from build123d import *

# Parameters (mm, degrees)
SKETCH1_W           = 84
SKETCH1_H           = 50.8
SKETCH1_R           = 2.1
BOSS_EXTRUDE1_DEPTH = 6
SKETCH3_W           = 20
SKETCH3_H           = 50.8
BOSS_EXTRUDE2_DEPTH = 20
SKETCH5_R           = 6.5
CUT_EXTRUDE1_DEPTH  = 10
CUT_EXTRUDE2_START  = -10
SKETCH6_R           = 6.5
CUT_EXTRUDE2_DEPTH  = 10
SKETCH7_W           = 10
SKETCH7_H           = 15
CUT_EXTRUDE3_DEPTH  = 10


with BuildPart() as part:
    # Sketch1 → Boss-Extrude1 (new body)
    with BuildSketch(Plane.XY):
        with Locations((42, 25.4)):
            Rectangle(SKETCH1_W, SKETCH1_H)
        with Locations((72, 39.4)):
            Circle(SKETCH1_R, mode=Mode.SUBTRACT)
        with Locations((72, 11.4)):
            Circle(SKETCH1_R, mode=Mode.SUBTRACT)
        with Locations((44, 39.4)):
            Circle(SKETCH1_R, mode=Mode.SUBTRACT)
        with Locations((44, 11.4)):
            Circle(SKETCH1_R, mode=Mode.SUBTRACT)
    extrude(amount=BOSS_EXTRUDE1_DEPTH)

    # Sketch3 → Boss-Extrude2 (add)
    with BuildSketch(Plane(origin=(0, 0, 0), x_dir=(-1, 0, 0), z_dir=(0, 0, -1))):
        with Locations((-10, 25.4)):
            Rectangle(SKETCH3_W, SKETCH3_H)
    extrude(amount=BOSS_EXTRUDE2_DEPTH)

    # Sketch5 → Cut-Extrude1 (cut)
    with BuildSketch(Plane(origin=(0, 50.8, 0), x_dir=(1, 0, 0), z_dir=(0, 1, 0))):
        with Locations(Location((10, 10, 0), (0, 0, 270))):
            Circle(SKETCH5_R)
    extrude(amount=-CUT_EXTRUDE1_DEPTH, mode=Mode.SUBTRACT)

    # Sketch6 → Cut-Extrude2 (cut)
    with BuildSketch(Plane.XZ.offset(CUT_EXTRUDE2_START)):
        with Locations(Location((10, -10, 0), (0, 0, 90))):
            Circle(SKETCH6_R)
    extrude(amount=CUT_EXTRUDE2_DEPTH, mode=Mode.SUBTRACT)

    # Sketch7 → Cut-Extrude3 (cut)
    with BuildSketch(Plane(origin=(0, 0, -20), x_dir=(-1, 0, 0), z_dir=(0, 0, -1))):
        with Locations((-15, 25.4)):
            Rectangle(SKETCH7_W, SKETCH7_H)
    extrude(amount=-CUT_EXTRUDE3_DEPTH, mode=Mode.SUBTRACT)


solid = part.part
For this review, take the finished solid that the model builds, in its own axes (mm). A direction names the side the tool comes from. Give positions to 0.01 mm unless a question says otherwise; leave off trailing zeros. Order: outer loops, then holes, each group sorted by start corner. A loop starts at its lowest first (then second) coordinate and runs counter-clockwise, first axis right, second up. Notation, with made-up numbers: M 87.25,75.5 L 105.25,75.5 A5 cw 105.25,83.5 Z; hole C 22.25,34.5 d1. An arc over 180 degrees is marked long. Answer in a Markdown table with one row per item. Add a question column.
(1) For pin 1 (4 mm diameter, centred on y = 26.5, z = -16, fed in from +X); pin 2 (15 mm diameter, centred on x = 41, y = 25.5, fed in from -Z); pin 3 (8 mm diameter, centred on y = 28.5, z = -12.5, fed in from +X), all flat-tipped, find the tip position at first contact; note any pin that passes through.
(2) Consider section A-A on y = 11.4. State the section outline as (x, z) points, and give its area (3 significant figures).
(3) For faces 4 (the face through (52, 26, 0)), 5 (the face through (10, 10, -10)), 6 (the face through (15, 26, -10)), 7 (the face through (71.54, 9.35, 2.96)), 8 (the face through (10, 40.8, -10)), list the 3-axis set-ups (+Z, -Z, +X, -X, +Y, -Y) from which the entire face can be reached by the end or side of a thin tool; tool diameter is ignored.
(4) Consider section D-D on z = -11.75. State the section outline as (x, y) points, and give its area (3 significant figures).
(5) Consider section B-B on x = 72. State the section outline as (y, z) points.
(6) Mouldability with a two-part tool opening along X and no side actions: class faces 1 (the face through (30, 0, 2)), 2 (the face through (71.727, 41.482, 2.958)), 3 (the face through (0, 25, -7)) as +X half, -X half, draft (parallel to the pull), parting line (faces both ways), or undercut.
(7) Wall thickness on probe 1 along Y at (x, z) = (72, 4.55); probe 2 along X at (y, z) = (5.5, -10); probe 3 along Y at (x, z) = (16, -16.5): over which ranges is each line inside the solid? List them lowest first. Write a range as [from, to].
(8) Consider section C-C on y = 4. State the section outline as (x, z) points, and give its area (3 significant figures).
Evaluation:
| question | item | result |
|---|---|---|
| 1 | pin 1 | stops at x = 10 |
| 1 | pin 2 | stops at z = 0 |
| 1 | pin 3 | stops at x = 20 |
| 2 | outline | M 0,-20 L 20,-20 L 20,0 L 41.9,0 L 41.9,6 L 0,6 Z; M 46.1,0 L 69.9,0 L 69.9,6 L 46.1,6 Z; M 74.1,0 L 84,0 L 84,6 L 74.1,6 Z |
| 2 | area | 854 mm^2 |
| 3 | face 4 | -Z, +X, +Y, -Y |
| 3 | face 5 | -Y |
| 3 | face 6 | -Z, +X |
| 3 | face 7 | +Z, -Z |
| 3 | face 8 | +Y |
| 4 | outline | M 0,0 L 3.74,0 L 3.74,10 L 16.26,10 L 16.26,0 L 20,0 L 20,17.9 L 10,17.9 L 10,32.9 L 20,32.9 L 20,50.8 L 16.26,50.8 L 16.26,40.8 L 3.74,40.8 L 3.74,50.8 L 0,50.8 Z |
| 4 | area | 616 mm^2 |
| 5 | outline | M 0,0 L 9.3,0 L 9.3,6 L 0,6 Z; M 13.5,0 L 37.3,0 L 37.3,6 L 13.5,6 Z; M 41.5,0 L 50.8,0 L 50.8,6 L 41.5,6 Z |
| 6 | face 1 | draft |
| 6 | face 2 | undercut |
| 6 | face 3 | -X half |
| 7 | probe 1 | y = [0, 9.3], [13.5, 37.3], [41.5, 50.8] |
| 7 | probe 2 | x = [0, 3.5], [16.5, 20] |
| 7 | probe 3 | y = [0, 17.9], [32.9, 50.8] |
| 8 | outline | M 0,-20 L 20,-20 L 20,0 L 84,0 L 84,6 L 0,6 Z; hole C 10,-10 d13 |
| 8 | area | 771 mm^2 |
